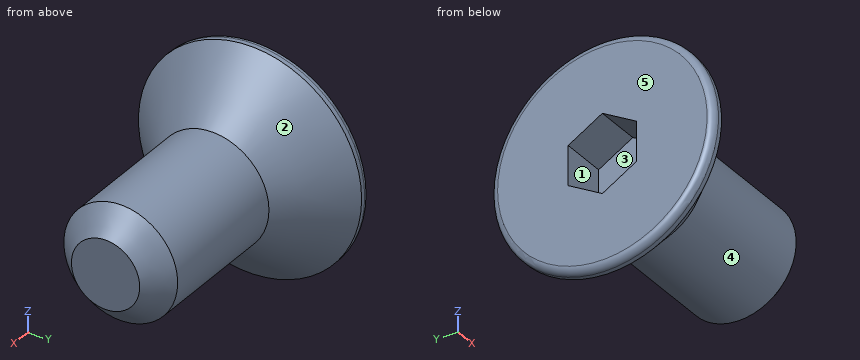
```python
from build123d import *

# Parameters (mm, degrees)
CUT_EXTRUDE_1_DEPTH = 2
FILLET_1_R          = 0.3
CHAMFER_1_SIZE      = 1


with BuildPart() as part:
    # Эскиз1 → Повернуть1 (revolve)
    with BuildSketch(Plane.XY):
        Polygon((0, 0), (0, 4.9), (0.5, 4.9), (3, 2.5), (10, 2.5), (10, 0), align=None)
    revolve(axis=Axis((10, 0, 0), (-1, 0, 0)))

    # Эскиз2 → Вырез-Вытянуть1 (cut)
    with BuildSketch(Plane.ZY):
        Polygon((0.866025404, 1.5), (-0.866025404, 1.5), (-1.732050808, 0), (-0.866025404, -1.5), (0.866025404, -1.5), (1.732050808, 0), align=None)
    extrude(amount=-CUT_EXTRUDE_1_DEPTH, mode=Mode.SUBTRACT)

    # Скругление1
    fillet_1_edges = [part.edges().sort_by_distance(p)[0] for p in [
        (0, -4.9, 0),
    ]]
    fillet(fillet_1_edges, radius=FILLET_1_R)

    # Фаска1
    chamfer_1_edges = [part.edges().sort_by_distance(p)[0] for p in [
        (10, -2.5, 0),
    ]]
    chamfer(chamfer_1_edges, length=CHAMFER_1_SIZE)


solid = part.part
```
Here's how the part is built. I have some questions about the finished solid (model axes, mm). Face numbers are marked on the shaded views. A direction names the side the tool comes from. Give positions to 0.01 mm unless a question says otherwise; leave off trailing zeros. Write each loop counter-clockwise with the first axis right and the second up, starting at its lowest first coordinate (ties: lowest second). Pieces come first, ordered by that corner, then holes.
(1) Imagine slicing it at A-A, the plane z = 0. Write out the boundary of the cut face in (x, y), and give its area (3 significant figures).
Output values:
outline: (0, -4.6) arc R0.3 ccw to (0.3, -4.9) - (0.5, -4.9) - (3, -2.5) - (9, -2.5) - (10, -1.5) - (10, 1.5) - (9, 2.5) - (3, 2.5) - (0.5, 4.9) - (0.3, 4.9) arc R0.3 ccw to (0, 4.6) - (0, 1.5) - (2, 1.5) - (2, -1.5) - (0, -1.5) - close
area: 51.4 mm2
(2) On a 3-axis mill with a long thin cutter (end or side, diameter ignored), from which of +Z, -Z, +X, -X, +Y, -Y can I reach the whole of each face in a straight line? I mean the marked faces 1 and 2. Say none if no direction works.
Output values:
face 1: -X
face 2: +X
(3) Imagine slicing it at C-C, the plane x = 6.5. Write out the boundary of the cut face in (y, z), and give its area (3 significant figures).
Output values:
outline: circle Ø5 at (0, 0)
area: 19.6 mm2
(4) Will these pins go through, and if not, where does the flat tip stop? pin 1 (0.9 mm diameter, centred on x = 1, z = -0.5, fed in from +Y); pin 2 (0.9 mm diameter, centred on x = 1.5, z = 0, fed in from -Y); pin 3 (5 mm diameter, centred on x = 5, y = 1, fed in from +Z).
Output values:
pin 1: stops at y = 4.83
pin 2: stops at y = -4.37
pin 3: stops at z = 2.89
(5) Thinking about a two-plate mould opening in Z: for the marked faces 3, 4 and 5, which applies, pulls with the +Z half, pulls with the -Z half, needs draft (parallel to the pull), parting line crosses it, or undercut?
Output values:
face 3: undercut
face 4: parting line crosses it
face 5: needs draft
(6) If I drill on L1, parallel to Y at x = 8.75, z = 0; L2, parallel to Z at x = 1, y = 1.25; L3, parallel to Y at x = 7.25, z = -1, over which ranges is the centre line in solid material (lowest first)?
Output values:
L1: y = -2.5 to 2.5
L2: z = -4.24 to -1.01, 1.01 to 4.24
L3: y = -2.29 to 2.29
(7) Imagine slicing it at B-B, the plane x = 2.75. Write out the boundary of the cut face in (y, z).
Output values:
outline: circle Ø5.48 at (0, 0)
